from build123d import *

# Parameters (mm, degrees)
F1_DEPTH     = 12.7
F2_T1_DEPTH  = 38.1
F2_T3_DEPTH  = 41.6542533238
F2_T5_DEPTH  = 41.5408544992
F2_T7_DEPTH  = 35.6725625774
F2_T9_DEPTH  = 33.4559034625
F2_T11_DEPTH = 42.4902813585
F2_T13_DEPTH = 46.0406969882


# Not quite as in the source:
# - a fillet or chamfer that OpenCascade refuses, or shapes differently, is made with other operations: its cross-section is extruded or revolved along the edge and cut away or added


with BuildPart() as f1:
    # F0 (on Front) → F1 (new body)
    with BuildSketch(Plane.XZ):
        with BuildLine():
            ThreePointArc((4.9426316758, 33.3698169468), (22.5960240749, 43.4449478875), (29.579706142, 62.5336542726))
            ThreePointArc((29.579706142, 62.5336542726), (-19.0887063851, 85.1296783474), (-4.9426316758, 33.3698169468))
            Line((-4.9426316758, 33.3698169468), (4.9426316758, 33.3698169468))
        make_face()
        with BuildLine():
            Line((4.9426316758, 33.3698169468), (-4.9426316758, 33.3698169468))
            ThreePointArc((-4.9426316758, 33.3698169468), (0, 32.9539481306), (4.9426316758, 33.3698169468))
        make_face()
        with BuildLine():
            ThreePointArc((4.9426316758, 33.3698169468), (0, 32.9539481306), (-4.9426316758, 33.3698169468))
            Line((-4.9426316758, 33.3698169468), (-4.9426316758, 27.7676489204))
            Line((-4.9426316758, 27.7676489204), (-4.9426316758, 17.8345050663))
            Line((-4.9426316758, 17.8345050663), (-4.9426316758, -32.282717526))
            Line((-4.9426316758, -32.282717526), (0.4634799664, -32.282717526))
            Line((0.4634799664, -32.282717526), (5.8695916086, -32.282717526))
            Line((5.8695916086, -32.282717526), (5.8695916086, 16.9314928353))
            Line((5.8695916086, 16.9314928353), (5.8695916086, 26.8646366894))
            Line((5.8695916086, 26.8646366894), (5.8695916086, 33.3698169468))
            Line((5.8695916086, 33.3698169468), (4.9426316758, 33.3698169468))
        make_face()
        Polygon((-4.9426316758, 17.8345050663), (-4.9426316758, 27.7676489204), (-39.732567966, 0), (-31.750221352, -10.0010386527), align=None)
        Polygon((40.6355895102, 0), (5.8695916086, 26.8646366894), (5.8695916086, 16.9314928353), (32.8805417262, -10.0359434636), align=None)
        Polygon((0.4634799664, -32.282717526), (-4.9426316758, -32.282717526), (-13.5451909155, -86.0119983554), (-4.9426316758, -86.0119983554), align=None)
        Polygon((5.8695916086, -32.282717526), (0.4634799664, -32.282717526), (5.8695916086, -86.0119983554), (15.1662486102, -86.9474057324), align=None)
    extrude(amount=F1_DEPTH)

    # F2: fillet of radius 5.08 on 8 edges, made by hand

    # F2_s2 → F2_t1 (cut)
    with BuildSketch(Plane.XZ.offset(-12.7)):
        with BuildLine():
            ThreePointArc((37.5294360638, -4.0197276981), (38.5484672449, -0.2675797032), (36.6158618121, 3.1061534464))
            Line((36.6158618121, 3.1061534464), (40.6355895102, 0))
            Line((40.6355895102, 0), (37.5294360638, -4.0197276981))
        make_face()
        with BuildLine():
            ThreePointArc((-35.7621773131, 3.168974292), (-37.641496387, -0.2347294175), (-36.5635936739, -3.9703906529))
            Line((-36.5635936739, -3.9703906529), (-39.732567966, 0))
            Line((-39.732567966, 0), (-35.7621773131, 3.168974292))
        make_face()
    extrude(amount=F2_T1_DEPTH, mode=Mode.SUBTRACT)

    # F2_s4 → F2_t3 (cut)
    with BuildSketch(Plane.XZ.offset(-14.4771266619)):
        with BuildLine():
            ThreePointArc((-35.3626341248, -5.4750663394), (-31.6283156718, -7.3806038383), (-27.7332133062, -5.8299958835))
            Line((-27.7332133062, -5.8299958835), (-31.750221352, -10.0010386527))
            Line((-31.750221352, -10.0010386527), (-35.3626341248, -5.4750663394))
        make_face()
    extrude(amount=F2_T3_DEPTH, mode=Mode.SUBTRACT)

    # F2_s6 → F2_t5 (cut)
    with BuildSketch(Plane.XZ.offset(-14.4204272496)):
        with BuildLine():
            ThreePointArc((28.7985423047, -5.960520019), (32.7134460909, -7.4350713917), (36.4074755687, -5.4716764688))
            Line((36.4074755687, -5.4716764688), (32.8805417262, -10.0359434636))
            Line((32.8805417262, -10.0359434636), (28.7985423047, -5.960520019))
        make_face()
    extrude(amount=F2_T5_DEPTH, mode=Mode.SUBTRACT)

    # F2_s8 → F2_t7 (cut)
    with BuildSketch(Plane.XZ.offset(-11.4862812887)):
        with BuildLine():
            ThreePointArc((-9.5371441912, -86.0119983554), (-6.1295888664, -84.699619184), (-4.4826652871, -81.4405679254))
            Line((-4.4826652871, -81.4405679254), (-4.9426316758, -86.0119983554))
            Line((-4.9426316758, -86.0119983554), (-9.5371441912, -86.0119983554))
        make_face()
    extrude(amount=F2_T7_DEPTH, mode=Mode.SUBTRACT)

    # F2_s10 → F2_t9 (cut)
    with BuildSketch(Plane.XZ.offset(-10.3779517312)):
        with BuildLine():
            ThreePointArc((5.4540081087, -81.8816725212), (6.9163845644, -84.9652053996), (9.9999174428, -86.4275818554))
            Line((9.9999174428, -86.4275818554), (5.8695916086, -86.0119983554))
            Line((5.8695916086, -86.0119983554), (5.4540081087, -81.8816725212))
        make_face()
    extrude(amount=F2_T9_DEPTH, mode=Mode.SUBTRACT)

    # F2_s12 → F2_t11 (cut)
    with BuildSketch(Plane.XZ.offset(-14.8951406792)):
        with BuildLine():
            ThreePointArc((-12.6032474685, -80.1288718839), (-11.452770586, -84.2279441623), (-7.5871346438, -86.0119983554))
            Line((-7.5871346438, -86.0119983554), (-13.5451909155, -86.0119983554))
            Line((-13.5451909155, -86.0119983554), (-12.6032474685, -80.1288718839))
        make_face()
    extrude(amount=F2_T11_DEPTH, mode=Mode.SUBTRACT)

    # F2_s14 → F2_t13 (cut)
    with BuildSketch(Plane.XZ.offset(-16.6703484941)):
        with BuildLine():
            ThreePointArc((8.5316088631, -86.2798441603), (12.7526164419, -84.6929586624), (14.0482707219, -80.3736542564))
            Line((14.0482707219, -80.3736542564), (15.1662486102, -86.9474057324))
            Line((15.1662486102, -86.9474057324), (8.5316088631, -86.2798441603))
        make_face()
    extrude(amount=F2_T13_DEPTH, mode=Mode.SUBTRACT)


solid = f1.part
Check sheet for the modelled part. Datum: model origin and axes. Units: mm. A direction names the side the tool comes from. Give positions to 0.01 mm unless a question says otherwise; leave off trailing zeros. Order: outer loops, then holes, each group sorted by start corner. A loop starts at its lowest first (then second) coordinate and runs counter-clockwise, first axis right, second up. Notation, with made-up numbers: M -0.75,-24.5 L 36.25,-24.5 A22 ccw 36.25,-11.5 Z; hole C 80,-38.75 d2. An arc over 180 degrees is marked long. Answer as CSV lines item,"result". Start each with the question number.
Item 1: Cross-section at A-A on y = -7.5. Enter the section's corners in (x, z), plus the area to 3 significant figures.
Item 2: Tool access check on faces 5 (the face through (17.17, -6.26, 5.65)), 6 (the face through (6.636, -6.261, -84.661)), 7 (the face through (5.87, -6, 30)). Record the directions out of +Z, -Z, +X, -X, +Y, -Y that give a thin tool (end or side, any length) a straight path to the whole face; none if there is none.
Item 3: Gauge pin test, flat ends, axial feed: P1, Ø7, axis at y = -3.5, z = 29, coming from the +X side; P2, Ø1.5, axis at y = -11, z = -19, coming from the -X side; P3, Ø1.5, axis at x = -14, y = -9, coming from the +Z side. Record the tip position at first contact, or that the pin passes through.
Item 4: Mould release check, pull along Z, two halves, no side actions. Record for faces 1 (the face through (-37.635, -6.261, -0.179)), 2 (the face through (-4.943, -6, -7)), 3 (the face through (0, 0, 24)), 4 (the face through (-5.813, -6.261, -84.387)): +Z half, -Z half, draft (parallel to the pull), parting line (faces both ways), or undercut.
Item 5: Cross-section at B-B on x = -21. Enter the section's corners in (y, z).
Item 6: Thickness scan on line 1 (Z direction, x = 17, y = -2.75); line 2 (X direction, y = -1.5, z = 8.5); line 3 (X direction, y = -5, z = -48). Record the ranges inside material, lowest first. Write a range as [from, to].
Item 7: Cross-section at C-C on z = 38. Enter the section's corners in (x, y), plus the area to 3 significant figures.
Item 8: Cross-section at D-D on x = 31.5. Enter the section's corners in (y, z), plus the area to 3 significant figures.
Established:
1,outline,"M -36.56,-3.97 L -35.36,-5.48 A5.08 ccw -27.73,-5.83 L -4.94,17.83 L -4.94,-32.28 L -12.6,-80.13 A5.08 ccw -8.56,-85.92 A5.08 ccw -4.48,-81.44 L 0.46,-32.28 L 5.45,-81.88 A5.08 ccw 9.27,-86.3 A5.08 ccw 14.05,-80.37 L 5.87,-32.28 L 5.87,16.93 L 28.8,-5.96 A5.08 ccw 36.41,-5.47 L 37.53,-4.02 A5.08 ccw 36.62,3.11 L 5.87,26.86 L 5.87,33.37 L 4.94,33.37 A29.58 ccw long -4.94,33.37 L -4.94,27.77 L -35.76,3.17 A5.08 ccw Z"
1,area,"5,010 mm^2"
2,face 5,"+Y, -Y"
2,face 6,"-Z, +Y, -Y"
2,face 7,"+X, +Y, -Y"
3,P1,"stops at x = 7.64"
3,P2,"stops at x = -4.94"
3,P3,"stops at z = 88.98"
4,face 1,"parting line"
4,face 2,"undercut"
4,face 3,"draft"
4,face 4,"-Z half"
5,outline,"M -12.7,1.16 L 0,1.16 L 0,14.95 L -12.7,14.95 Z; M -12.7,41.7 L 0,41.7 L 0,83.37 L -12.7,83.37 Z"
6,line 1,"z = [5.82, 18.26], [38.33, 86.74]"
6,line 2,"x = [-29.08, -13.93], [-4.94, 5.87], [14.31, 29.64]"
6,line 3,"x = [-7.46, -1.12], [2.04, 8.54]"
7,outline,"M -16.52,-12.7 L 16.52,-12.7 L 16.52,0 L -16.52,0 Z"
7,area,"420 mm^2"
8,outline,"M -12.7,-7.37 L 0,-7.37 L 0,7.06 L -12.7,7.06 Z"
8,area,"183 mm^2"
